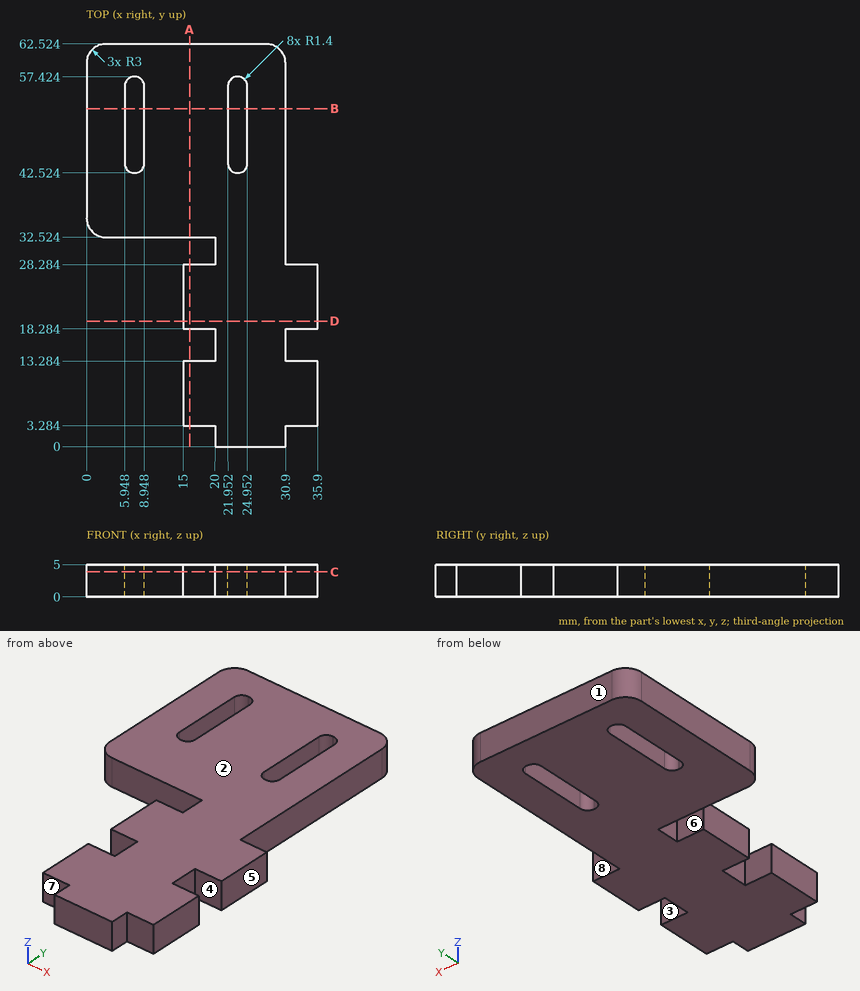
For this review, use the dimensioned drawing (mm, ordinates from the lowest corner) and the shaded views. A direction names the side the tool comes from. Coordinates: 2 decimals unless noted, no trailing zeros. Order: outer loops, then holes, each group sorted by start corner. A loop starts at its lowest first (then second) coordinate and runs counter-clockwise, first axis right, second up. Notation, with made-up numbers: M 20,80 L 34,80 A30 cw 34,102 Z; hole C 18,-15 d10. An arc over 180 degrees is marked long. Answer as a JSON object with one key per item and string values. Group by question number.
1) Tool access review of the marked faces 4, 5, 6, 7 and 8: name each direction out of +Z, -Z, +X, -X, +Y, -Y from which nothing blocks a thin tool from reaching the whole face with its end or side.
2) Add section C-C, the plane z = 3.9. Count the separate pieces of the cut face and the enclosed holes in it, then the cut area to 3 significant figures.
3) Add section B-B, the plane y = 52.5. Write out the cut boundary in (x, z).
4) Add section D-D, the plane y = 19.5. Write out the cut boundary in (x, z).
5) For pin 1 (2.5 mm diameter, centred on y = 2, z = 3, fed in from -X); pin 2 (1 mm diameter, centred on y = 1.5, z = 3.5, fed in from +X); pin 3 (2.5 mm diameter, centred on x = 33, z = 1.5, fed in from +Y), all flat-tipped, find the tip position at first contact; note any pin that passes through.
6) Wall thickness on L1, parallel to Y at x = 16.5, z = 1.7; L2, parallel to X at y = 46.5, z = 2.9; L3, parallel to Y at x = 34, z = 0.95: over which ranges is each line inside the solid? List them lowest first.
7) Mouldability with a two-part tool opening along Y and no side actions: class the marked faces 1, 2 and 3 as pulls with the +Y half, pulls with the -Y half, needs draft (parallel to the pull), parting line crosses it, or undercut.
8) Add section A-A, the plane x = 16. Write out the cut boundary in (y, z), then the cut area to 3 significant figures.
Computed values:
{
 "1": {"face 4": "+Z, -Z, +X", "face 5": "+Z, -Z, +X, +Y, -Y", "face 6": "+Z, -Z, -X", "face 7": "+Z, -Z, -X, -Y", "face 8": "+Z, -Z, +X, +Y"},
 "2": {"separate pieces": "1", "enclosed holes": "2", "area": "1,390 mm^2"},
 "3": {"outline": "M 0,0 L 5.95,0 L 5.95,5 L 0,5 Z; M 8.95,0 L 21.95,0 L 21.95,5 L 8.95,5 Z; M 24.95,0 L 30.9,0 L 30.9,5 L 24.95,5 Z"},
 "4": {"outline": "M 15,0 L 35.9,0 L 35.9,5 L 15,5 Z"},
 "5": {"pin 1": "stops at x = 20", "pin 2": "stops at x = 30.9", "pin 3": "stops at y = 28.28"},
 "6": {"L1": "y = 3.28 to 13.28, 18.28 to 28.28, 32.52 to 62.52", "L2": "x = 0 to 5.95, 8.95 to 21.95, 24.95 to 30.9", "L3": "y = 3.28 to 13.28, 18.28 to 28.28"},
 "7": {"face 1": "pulls with the +Y half", "face 2": "needs draft", "face 3": "undercut"},
 "8": {"outline": "M 3.28,0 L 13.28,0 L 13.28,5 L 3.28,5 Z; M 18.28,0 L 28.28,0 L 28.28,5 L 18.28,5 Z; M 32.52,0 L 62.52,0 L 62.52,5 L 32.52,5 Z", "area": "250 mm^2"}
}
